Source: three-view drawing plus pictorial views. Frame: mm from the lowest corner of the part. Give positions to 0.01 mm unless a question says otherwise; leave off trailing zeros. Write each loop counter-clockwise with the first axis right and the second up, starting at its lowest first coordinate (ties: lowest second). Pieces come first, ordered by that corner, then holes. Notation, with made-up numbers: (41.5, 25.5) -> (79.5, 25.5) arc R12 ccw to (79.5, 36.5) -> close; hole circle Ø6 at (5, -8). An arc over 180 degrees is marked (long way). Answer in a Markdown table with one row per item. Add a question column.
Item 1: Material intervals for probe 1 along Y at (x, z) = (1.85, 28.5) (1 decimal); probe 2 along Y at (x, z) = (2.95, 8.5) (1 decimal); probe 3 along Y at (x, z) = (0.25, 7.5) (1 decimal), sorted ascending. Write a range as from..to.
Item 2: Section query B-B on y = 12.25. Output: boundary loops of the cut face in (x, z) (1 decimal).
Item 3: Section query C-C on x = 0.8. State how many separate pieces and enclosed holes the cut face has, plus the area to 3 significant figures.
Item 4: Section query A-A on z = 6.35. Output: boundary loops of the cut face in (x, y) (1 decimal).
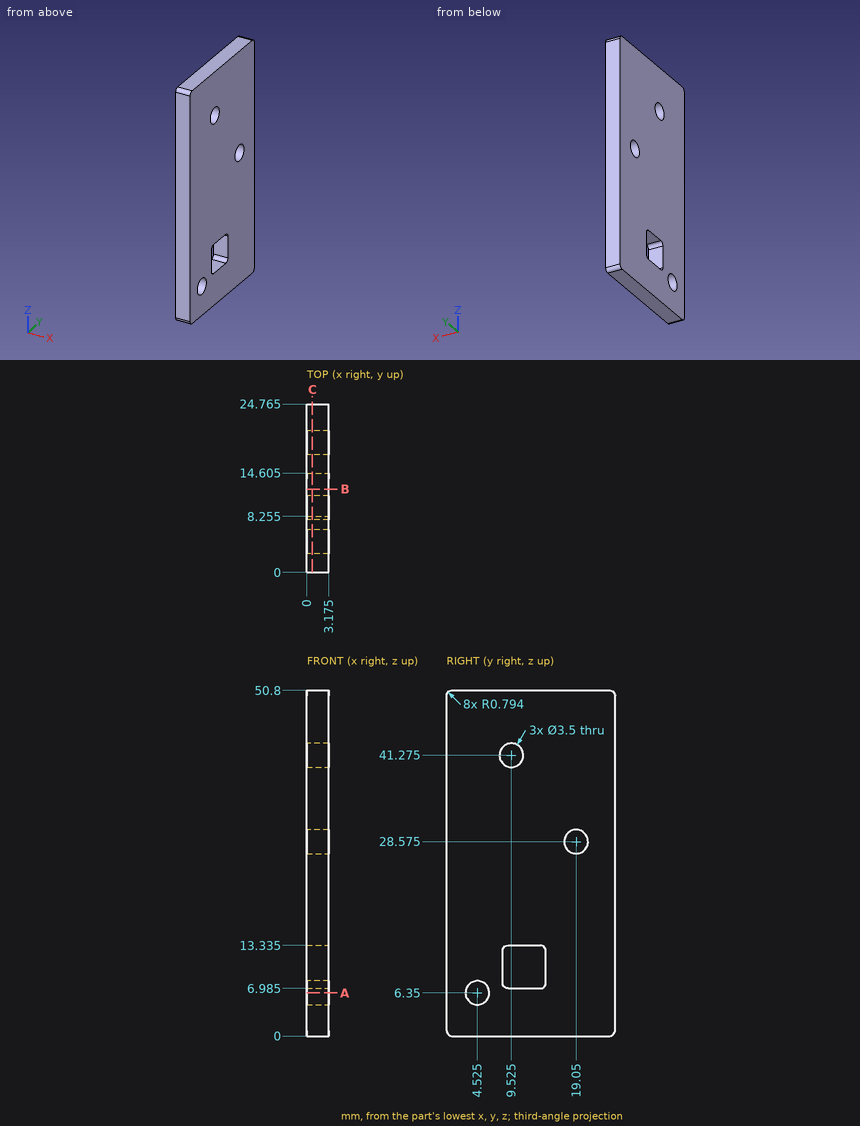
Findings below:
| question | item | result |
|---|---|---|
| 1 | probe 1 | y = 0..17.3, 20.8..24.8 |
| 1 | probe 2 | y = 0..8.3, 14.6..24.8 |
| 1 | probe 3 | y = 0..3.2, 5.8..8.3, 14.6..24.8 |
| 2 | outline | (0, 0) -> (3.2, 0) -> (3.2, 7) -> (0, 7) -> close; (0, 13.3) -> (3.2, 13.3) -> (3.2, 50.8) -> (0, 50.8) -> close |
| 3 | separate pieces | 1 |
| 3 | enclosed holes | 4 |
| 3 | area | 1,190 mm^2 |
| 4 | outline | (0, 0) -> (3.2, 0) -> (3.2, 2.8) -> (0, 2.8) -> close; (0, 6.3) -> (3.2, 6.3) -> (3.2, 24.8) -> (0, 24.8) -> close |
